Can you work these out from the model? Positions are in its coordinate system, mm. Face numbers are marked on the shaded views. Give positions to 0.01 mm unless a question says otherwise; leave off trailing zeros. Order: outer loops, then holes, each group sorted by start corner. A loop starts at its lowest first (then second) coordinate and runs counter-clockwise, first axis right, second up. Notation, with made-up numbers: M -27,2.25 L 10,2.25 A23 ccw 10,19.25 Z; hole C 60,0 d5. An arc over 180 degrees is marked long. Answer as a JSON object with one key per item and string values.
```python
from build123d import *

# Parameters (mm, degrees)
SKETCH1_R           = 63.5
BOSS_EXTRUDE1_DEPTH = 6.35
CUT_EXTRUDE1_DEPTH  = 91.02678768
SKETCH4_R           = 4.445
BOSS_EXTRUDE2_DEPTH = 15.875
CHAMFER2_SIZE       = 2.159
CHAMFER3_SIZE       = 1.5875


with BuildPart() as part:
    # Sketch1 → Boss-Extrude1 (new body)
    with BuildSketch(Plane.XY):
        Circle(SKETCH1_R)
    extrude(amount=BOSS_EXTRUDE1_DEPTH)

    # Sketch3 → Cut-Extrude1 (cut, through all)
    with BuildSketch(Plane.XY.offset(6.35)):
        with BuildLine():
            Line((-1.322875656, 1.5), (1.322875656, 1.5))
            ThreePointArc((1.322875656, 1.5), (0, -2), (-1.322875656, 1.5))
        make_face()
    extrude(amount=-CUT_EXTRUDE1_DEPTH, mode=Mode.SUBTRACT)

    # Sketch4 → Boss-Extrude2 (add)
    with BuildSketch(Plane.XY.offset(6.35)):
        with Locations((0, 19.05)):
            Circle(SKETCH4_R)
    boss_extrude2 = extrude(amount=BOSS_EXTRUDE2_DEPTH)

    # Mirror3: Boss-Extrude2 across plane
    add(boss_extrude2.mirror(Plane.ZX))

    # Chamfer2
    chamfer2_edges = [part.edges().sort_by_distance(p)[0] for p in [
        (-4.445, 19.05, 22.225),
        (-4.445, -19.05, 22.225),
    ]]
    chamfer(chamfer2_edges, length=CHAMFER2_SIZE)

    # Chamfer3
    chamfer3_edges = [part.edges().sort_by_distance(p)[0] for p in [
        (-4.445, 19.05, 6.35),
        (-4.445, -19.05, 6.35),
    ]]
    chamfer(chamfer3_edges, length=CHAMFER3_SIZE)


solid = part.part
```
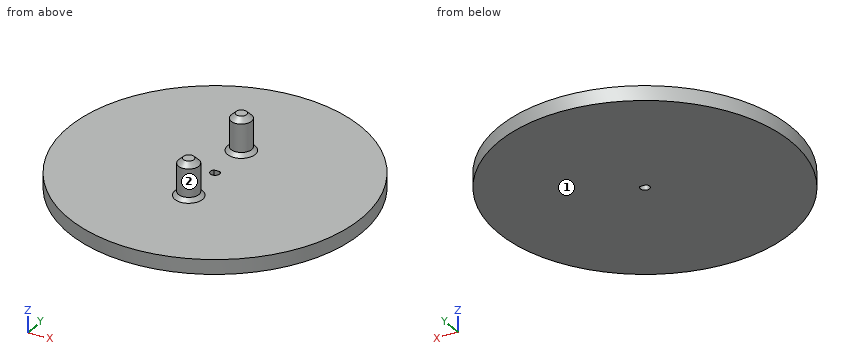
1) I want a section at B-B on z = 14. Write out the boundary of the cut face in (x, y) (3 decimals).
Results found:
{"outline": "C 0,-19.05 d8.89; C 0,19.05 d8.89"}
2) I'm going to push flat-ended pins straight in: pin 1 Ø12 at (x, z) = (5.5, 17) entering from +Y (3 decimals); pin 2 Ø6 at (x, y) = (1, 1) entering from +Z; pin 3 Ø0.8 at (x, z) = (0.5, 3.5) entering from -Y. Where does each tip first touch, or does it pass through?
Results found:
{"pin 1": "stops at y = 23.495", "pin 2": "stops at z = 6.35", "pin 3": "stops at y = -63.5"}
3) Thinking about a two-plate mould opening in Y: for the marked faces 1 and 2, which applies, pulls with the +Y half, pulls with the -Y half, needs draft (parallel to the pull), parting line crosses it, or undercut?
Results found:
{"face 1": "needs draft", "face 2": "undercut"}
4) I want a section at A-A on y = 0. Write out the boundary of the cut face in (x, z), and give its area (3 significant figures).
Results found:
{"outline": "M -63.5,0 L -2,0 L -2,6.35 L -63.5,6.35 Z; M 2,0 L 63.5,0 L 63.5,6.35 L 2,6.35 Z", "area": "781 mm²"}
5) I need wall thicknesses on L1, parallel to Z at x = 40, y = -48.5; L2, parallel to Y at x = 49, z = 3; L3, parallel to X at y = 54, z = 4. Which ranges of each line are inside material? Lowest first, please.
Results found:
{"L1": "z = 0 to 6.35", "L2": "y = -40.39 to 40.39", "L3": "x = -33.41 to 33.41"}
6) I want a section at D-D on x = -9.5. Write out the boundary of the cut face in (y, z).
Results found:
{"outline": "M -62.79,0 L 62.79,0 L 62.79,6.35 L -62.79,6.35 Z"}
